Read the model definition and answer for the solid it produces. Units are mm, in the model's axes. Face numbers are marked on the shaded views. Give positions to 0.01 mm unless a question says otherwise; leave off trailing zeros. Write each loop counter-clockwise with the first axis right and the second up, starting at its lowest first coordinate (ties: lowest second). Pieces come first, ordered by that corner, then holes. Notation, with made-up numbers: (68.25, 73) -> (75.25, 73) arc R22 ccw to (75.25, 106) -> close; hole circle Ø2 at (76, 28.5). An arc over 180 degrees is marked (long way). Write item = value, one per line.
from build123d import *

# Parameters (mm, degrees)
F2_R    = 5.08
F3_SIZE = 2.54
F4_SIZE = 2.54


with BuildPart() as f1:
    # F0 (on Front) → F1 (revolve)
    with BuildSketch(Plane.XZ):
        Polygon((-42.06875, 0), (-29.36875, 0), (-29.36875, -19.05), (-16.66875, -19.05), (-16.66875, 6.35), (-42.06875, 6.35), align=None)
    revolve(axis=Axis((0, 0, -9.525), (0, 0, -1)))

    # F2
    f2_edges = [f1.edges().sort_by_distance(p)[0] for p in [
        (42.06875, 0, 6.35),
    ]]
    fillet(f2_edges, radius=F2_R)

    # F3
    f3_edges = [f1.edges().sort_by_distance(p)[0] for p in [
        (16.66875, 0, 6.35),
    ]]
    chamfer(f3_edges, length=F3_SIZE)

    # F4
    f4_edges = [f1.edges().sort_by_distance(p)[0] for p in [
        (29.36875, 0, -19.05),
    ]]
    chamfer(f4_edges, length=F4_SIZE)


solid = f1.part
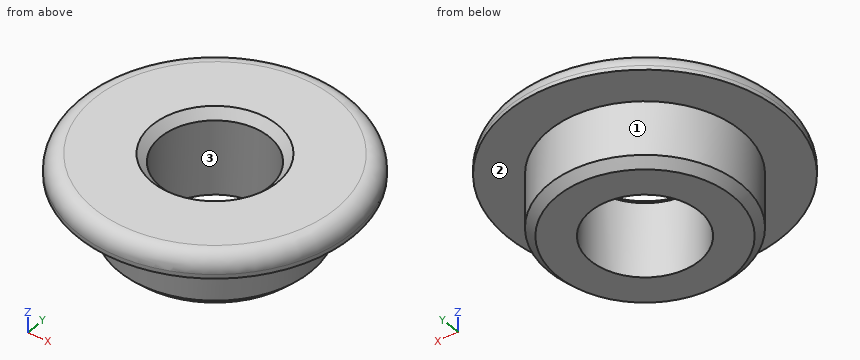
(1) For a pull along Y with two mould halves and no side action, classify the marked faces 1, 2 and 3 as released by +Y, released by -Y, zero draft, split by the parting line, or undercut.
Checks:
face_1 = split by the parting line
face_2 = zero draft
face_3 = undercut
(2) The part is cut by section A-A on y = 0. Determine the outline of the cut face in (x, z).
Checks:
outline = (-42.07, 0) -> (-29.37, 0) -> (-29.37, -16.51) -> (-26.83, -19.05) -> (-16.67, -19.05) -> (-16.67, 3.81) -> (-19.21, 6.35) -> (-36.99, 6.35) arc R5.08 ccw to (-42.07, 1.27) -> close; (16.67, -19.05) -> (26.83, -19.05) -> (29.37, -16.51) -> (29.37, 0) -> (42.07, 0) -> (42.07, 1.27) arc R5.08 ccw to (36.99, 6.35) -> (19.21, 6.35) -> (16.67, 3.81) -> close
(3) The part is cut by section C-C on z = -13.5. Determine the outline of the cut face in (x, y), plus the area to 3 significant figures.
Checks:
outline = circle Ø58.74 at (0, 0); hole circle Ø33.34 at (0, 0)
area = 1,840 mm²
(4) Consider L1, parallel to Y at x = 0, z = -3.5; L2, parallel to X at y = -4.5, z = -4; L3, parallel to X at y = -15, z = -4.75. Determine where each line is inside the solid, lowest interval first.
Checks:
L1 = -29.37 to -16.67, 16.67 to 29.37
L2 = -29.02 to -16.05, 16.05 to 29.02
L3 = -25.25 to -7.27, 7.27 to 25.25
(5) Given P1, Ø20, axis at x = 0, y = 0, coming from the +Z side; P2, Ø8, axis at y = 31, z = -9.5, coming from the -X side; P3, Ø1, axis at x = 11, z = -4.5, coming from the +Y side; P4, Ø6, axis at x = 28, z = -0.5, coming from the -Y side, each flat-ended and moving along its own axis, determine where each tip first touches the part or whether it passes through.
Checks:
P1 = through
P2 = -11.56
P3 = 27.43
P4 = -33.8
